Could you check a few things on this drawing? It's one solid part, dimensions in mm from its lowest x, y, z. Give positions to 0.01 mm unless a question says otherwise; leave off trailing zeros. Loops run counter-clockwise (first coordinate to the right, second up) from the corner with the lowest first, then second, coordinate; pieces in that order, holes last. Notation, with made-up numbers: (22.25, 87) - (71.25, 87) arc R19 ccw to (71.25, 97) - close; hole circle Ø5 at (71.5, 86.5). An arc over 180 degrees is marked (long way). Write item = value, one per line.
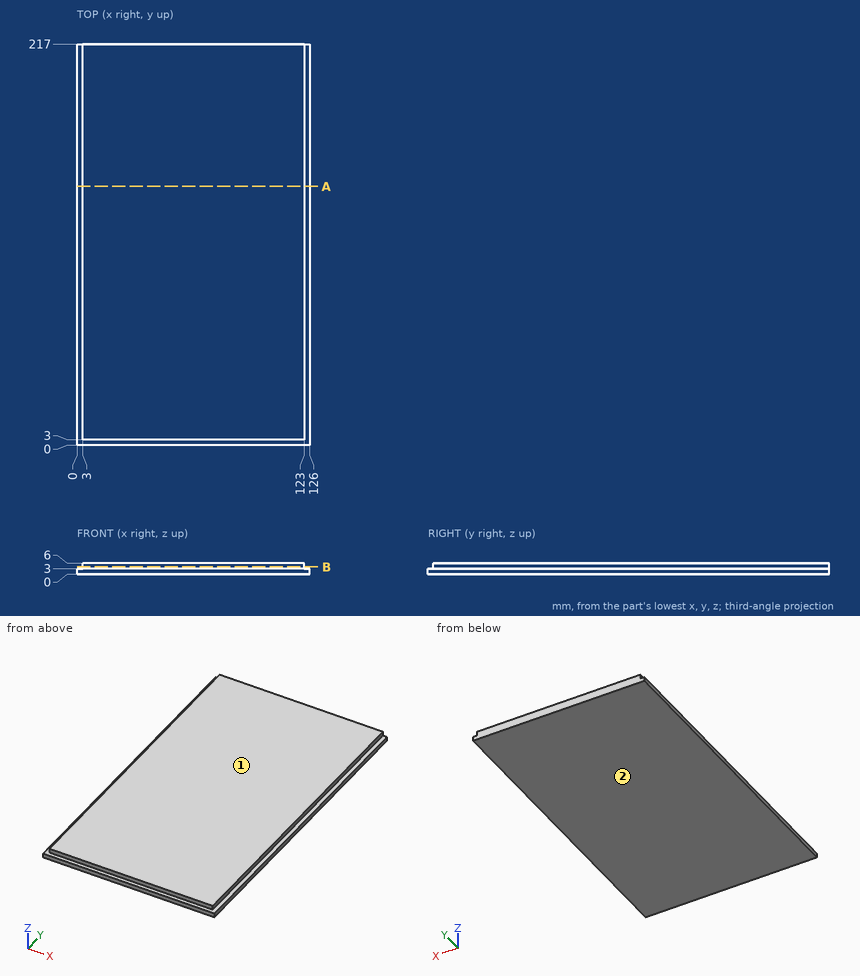
Q1. I need wall thicknesses on L1, parallel to Y at x = 98.5, z = 5.1; L2, parallel to X at y = 69, z = 4.6. Which ranges of each line are inside material? Lowest first, please.
Output:
L1 = 3 to 217
L2 = 3 to 123
Q2. Imagine slicing it at B-B, the plane z = 3.95. Write out the boundary of the cut face in (x, y), then the cut area to 3 significant figures.
Output:
outline = (3, 3) - (123, 3) - (123, 217) - (3, 217) - close
area = 25,700 mm2
Q3. For pin 1 (2.5 mm diameter, centred on y = 154.5, z = 5, fed in from -X); pin 2 (1.5 mm diameter, centred on x = 88, z = 5, fed in from -Y), each with a flat end and sliding along its axis, tell me the tip position at first contact or that it passes through.
Output:
pin_1 = 3
pin_2 = 3
Q4. We'd pull the mould along Z, two halves only. Please class the marked faces 1 and 2: released by +Z, released by -Z, zero draft, split by the parting line, or undercut.
Output:
face_1 = released by +Z
face_2 = released by -Z
Q5. Imagine slicing it at A-A, the plane y = 140. Write out the boundary of the cut face in (x, z), then the cut area to 3 significant figures.
Output:
outline = (0, 0) - (126, 0) - (126, 3) - (123, 3) - (123, 6) - (3, 6) - (3, 3) - (0, 3) - close
area = 738 mm2
